```python
from build123d import *

# Parameters (mm, degrees)
SKETCH1_W           = 270
SKETCH1_H           = 60
BOSS_EXTRUDE1_DEPTH = 2
SKETCH6_W           = 270
SKETCH6_H           = 5.6
BOSS_EXTRUDE2_DEPTH = 2
SKETCH7_R           = 2.5
SKETCH7_R_2         = 3
CUT_EXTRUDE1_DEPTH  = 140.629366539
SKETCH8_W           = 90
SKETCH8_H           = 10
CUT_EXTRUDE2_DEPTH  = 140.629366539
SKETCH9_R           = 29
CUT_EXTRUDE3_DEPTH  = 10
SKETCH10_R          = 1.0668
CUT_EXTRUDE4_DEPTH  = 10
SKETCH11_W          = 90
SKETCH11_H          = 9
CUT_EXTRUDE5_DEPTH  = 10


with BuildPart() as part:
    # Sketch1 → Boss-Extrude1 (new body)
    with BuildSketch(Plane.XY):
        Rectangle(SKETCH1_W, SKETCH1_H)
    extrude(amount=BOSS_EXTRUDE1_DEPTH)

    # Sketch6 → Boss-Extrude2 (add)
    with BuildSketch(Plane.XY.offset(2)):
        with Locations((0, 32.8)):
            Rectangle(SKETCH6_W, SKETCH6_H)
    extrude(amount=-BOSS_EXTRUDE2_DEPTH)

    # Sketch7 → Cut-Extrude1 (cut, through all)
    with BuildSketch(Plane(origin=(0, 0, 0), x_dir=(-1, 0, 0), z_dir=(0, 0, -1))):
        with Locations((-36.5, 20.124709067)):
            Circle(SKETCH7_R)
        with Locations((-36.5, -9.875290933)):
            Circle(SKETCH7_R)
        with Locations((36.5, -9.875290933)):
            Circle(SKETCH7_R)
        with Locations((36.5, 20.124709067)):
            Circle(SKETCH7_R)
        with Locations((125, 24)):
            Circle(SKETCH7_R_2)
        with Locations((120, -24)):
            Circle(SKETCH7_R_2)
        with Locations((-125, 24)):
            Circle(SKETCH7_R_2)
        with Locations((-120, -24)):
            Circle(SKETCH7_R_2)
    extrude(amount=-CUT_EXTRUDE1_DEPTH, mode=Mode.SUBTRACT)

    # Sketch8 → Cut-Extrude2 (cut, through all)
    with BuildSketch(Plane(origin=(0, 0, 0), x_dir=(-1, 0, 0), z_dir=(0, 0, -1))):
        with Locations((-90, 9.6)):
            Rectangle(SKETCH8_W, SKETCH8_H)
    extrude(amount=-CUT_EXTRUDE2_DEPTH, mode=Mode.SUBTRACT)

    # Sketch9 → Cut-Extrude3 (cut)
    with BuildSketch(Plane.XY.offset(2)):
        with Locations((-94, 2.8)):
            Circle(SKETCH9_R)
    extrude(amount=-CUT_EXTRUDE3_DEPTH, mode=Mode.SUBTRACT)

    # Sketch10 → Cut-Extrude4 (cut)
    with BuildSketch(Plane(origin=(0, 0, 0), x_dir=(-1, 0, 0), z_dir=(0, 0, -1))):
        with Locations((56.3119, -22.5108)):
            Circle(SKETCH10_R)
        with Locations((56.3119, 5.0228)):
            Circle(SKETCH10_R)
        with BuildLine():
            Line((62.6238, -19.793), (62.6238, 2.305))
            ThreePointArc((62.6238, 2.305), (62.512207684, 2.574407684), (62.2428, 2.686))
            Line((62.2428, 2.686), (50.381, 2.686))
            ThreePointArc((50.381, 2.686), (50.111592316, 2.574407684), (50, 2.305))
            Line((50, 2.305), (50, -19.793))
            ThreePointArc((50, -19.793), (50.111592316, -20.062407684), (50.381, -20.174))
            Line((50.381, -20.174), (62.2428, -20.174))
            ThreePointArc((62.2428, -20.174), (62.512207684, -20.062407684), (62.6238, -19.793))
        make_face()
    extrude(amount=-CUT_EXTRUDE4_DEPTH, mode=Mode.SUBTRACT)

    # Sketch11 → Cut-Extrude5 (cut)
    with BuildSketch(Plane.XY.offset(2)):
        with Locations((90, 0.1)):
            Rectangle(SKETCH11_W, SKETCH11_H)
    extrude(amount=-CUT_EXTRUDE5_DEPTH, mode=Mode.SUBTRACT)


solid = part.part
```
Verification items for the finished model (mm, model axes). Round coordinates to 2 decimals unless told otherwise and drop trailing zeros. Loops run counter-clockwise (first coordinate to the right, second up) from the corner with the lowest first, then second, coordinate; pieces in that order, holes last. Notation, with made-up numbers: (87.25, -39.5) -> (140.25, -39.5) arc R29 ccw to (140.25, -7.5) -> close; hole circle Ø1 at (66, 24). An arc over 180 degrees is marked (long way). Answer as a JSON object with one key per item and string values.
Q1. Section check A-A (x = -36.5). Record the boundary of the cut face in (y, z).
Data:
{"outline": "(-30, 0) -> (-12.38, 0) -> (-12.38, 2) -> (-30, 2) -> close; (-7.38, 0) -> (17.62, 0) -> (17.62, 2) -> (-7.38, 2) -> close; (22.62, 0) -> (35.6, 0) -> (35.6, 2) -> (22.62, 2) -> close"}
Q2. Scan lines: line 1 (Y direction, x = 125, z = 1.05); line 2 (Y direction, x = 38, z = 0.4); line 3 (Y direction, x = -60.5, z = 1.6). Record each from-to range of solid material in increasing order. Write a range as from..to.
Data:
{"line 1": "y = -30..-4.4, 14.6..21, 27..35.6", "line 2": "y = -30..-11.88, -7.88..18.12, 22.12..35.6", "line 3": "y = -30..-20.17, 2.69..35.6"}
Q3. Go/stop test with a flat-tipped pin: P1, Ø1, axis at y = 0.5, z = 0.5, coming from the +X side. Record where the tip stops, or that it passes through.
Data:
{"P1": "stops at x = 45"}
Q4. Section check D-D (z = 0.7). State how many separate pieces and enclosed holes the cut face has, then the cut area to 3 significant figures.
Data:
{"separate pieces": "1", "enclosed holes": "12", "area": "12,900 mm2"}
Q5. Section check C-C (y = 0). Record the boundary of the cut face in (x, z), then the cut area to 3 significant figures.
Data:
{"outline": "(-135, 0) -> (-122.86, 0) -> (-122.86, 2) -> (-135, 2) -> close; (-65.14, 0) -> (-62.62, 0) -> (-62.62, 2) -> (-65.14, 2) -> close; (-50, 0) -> (45, 0) -> (45, 2) -> (-50, 2) -> close", "area": "219 mm2"}
Q6. Draft check along X on faces 1 (the cylindrical face through (122.14, 24.9, 0.99)), 2 (the cylindrical face through (-122.97, 4.08, 1.01)), 3 (the flat face through (-2, 3, 2)). Enter one of: pulls with the +X half, pulls with the -X half, needs draft (parallel to the pull), parting line crosses it, or undercut.
Data:
{"face 1": "undercut", "face 2": "undercut", "face 3": "needs draft"}
Q7. Section check B-B (x = 62). Record the boundary of the cut face in (y, z), then the cut area to 3 significant figures.
Data:
{"outline": "(-30, 0) -> (-4.4, 0) -> (-4.4, 2) -> (-30, 2) -> close; (14.6, 0) -> (35.6, 0) -> (35.6, 2) -> (14.6, 2) -> close", "area": "93.2 mm2"}
